The listing builds one solid part. Answer for the finished solid, in the listing's coordinates (mm). Round coordinates to 2 decimals unless told otherwise and drop trailing zeros. Loops run counter-clockwise (first coordinate to the right, second up) from the corner with the lowest first, then second, coordinate; pieces in that order, holes last. Notation, with made-up numbers: (-2.75, 47) -> (11.25, 47) arc R23 ccw to (11.25, 62) -> close; hole circle Ø8 at (27.25, -17.5). An arc over 180 degrees is marked (long way). Answer in a Markdown table with one row per item. Add a question column.
```python
from build123d import *

# Parameters (mm, degrees)
SKETCH_2_R      = 1.75
SKETCH_2_W      = 27.3
SKETCH_2_H      = 20.5
SKETCH_2_W_2    = 9
SKETCH_2_H_2    = 14
EXTRUDE_1_DEPTH = 1.6


with BuildPart() as part:
    # 草图2 → 凸台-拉伸1 (new body)
    with BuildSketch(Plane.XY):
        with BuildLine():
            Line((137.6194709, 153.362234659), (251.6194709, 153.362234659))
            ThreePointArc((251.6194709, 153.362234659), (253.740791244, 152.483555002), (254.6194709, 150.362234659))
            Line((254.6194709, 150.362234659), (254.6194709, 97.362234659))
            ThreePointArc((254.6194709, 97.362234659), (253.740791244, 95.240914315), (251.6194709, 94.362234659))
            Line((251.6194709, 94.362234659), (137.6194709, 94.362234659))
            ThreePointArc((137.6194709, 94.362234659), (135.498150556, 95.240914315), (134.6194709, 97.362234659))
            Line((134.6194709, 97.362234659), (134.6194709, 150.362234659))
            ThreePointArc((134.6194709, 150.362234659), (135.498150556, 152.483555002), (137.6194709, 153.362234659))
        make_face()
        with Locations((139.6194709, 99.362234659)):
            Circle(SKETCH_2_R, mode=Mode.SUBTRACT)
        with Locations((249.6194709, 99.362234659)):
            Circle(SKETCH_2_R, mode=Mode.SUBTRACT)
        with Locations((249.6194709, 148.362234659)):
            Circle(SKETCH_2_R, mode=Mode.SUBTRACT)
        with Locations((139.6194709, 148.362234659)):
            Circle(SKETCH_2_R, mode=Mode.SUBTRACT)
        with Locations((173.2694709, 135.112234659)):
            Rectangle(SKETCH_2_W, SKETCH_2_H, mode=Mode.SUBTRACT)
        with BuildLine():
            Line((211.624069471, 144.588100568), (235.624069471, 144.588100568))
            ThreePointArc((235.624069471, 144.588100568), (236.874069471, 143.338100568), (235.624069471, 142.088100568))
            Line((235.624069471, 142.088100568), (211.624069471, 142.088100568))
            ThreePointArc((211.624069471, 142.088100568), (210.374069471, 143.338100568), (211.624069471, 144.588100568))
        make_face(mode=Mode.SUBTRACT)
        with BuildLine():
            Line((212.067868177, 135.739898553), (236.067868177, 135.739898553))
            ThreePointArc((236.067868177, 135.739898553), (237.317868177, 134.489898553), (236.067868177, 133.239898553))
            Line((236.067868177, 133.239898553), (212.067868177, 133.239898553))
            ThreePointArc((212.067868177, 133.239898553), (210.817868177, 134.489898553), (212.067868177, 135.739898553))
        make_face(mode=Mode.SUBTRACT)
        with BuildLine():
            Line((212.536781854, 118.268660205), (236.536781854, 118.268660205))
            ThreePointArc((236.536781854, 118.268660205), (237.786781854, 117.018660205), (236.536781854, 115.768660205))
            Line((236.536781854, 115.768660205), (212.536781854, 115.768660205))
            ThreePointArc((212.536781854, 115.768660205), (211.286781854, 117.018660205), (212.536781854, 118.268660205))
        make_face(mode=Mode.SUBTRACT)
        with BuildLine():
            Line((150.12910228, 109.191368081), (174.12910228, 109.191368081))
            ThreePointArc((174.12910228, 109.191368081), (175.37910228, 107.941368081), (174.12910228, 106.691368081))
            Line((174.12910228, 106.691368081), (150.12910228, 106.691368081))
            ThreePointArc((150.12910228, 106.691368081), (148.87910228, 107.941368081), (150.12910228, 109.191368081))
        make_face(mode=Mode.SUBTRACT)
        with BuildLine():
            Line((181.33094074, 109.046397883), (205.33094074, 109.046397883))
            ThreePointArc((205.33094074, 109.046397883), (206.58094074, 107.796397883), (205.33094074, 106.546397883))
            Line((205.33094074, 106.546397883), (181.33094074, 106.546397883))
            ThreePointArc((181.33094074, 106.546397883), (180.08094074, 107.796397883), (181.33094074, 109.046397883))
        make_face(mode=Mode.SUBTRACT)
        with BuildLine():
            Line((217.663513674, 108.782143694), (241.663513674, 108.782143694))
            ThreePointArc((241.663513674, 108.782143694), (242.913513674, 107.532143694), (241.663513674, 106.282143694))
            Line((241.663513674, 106.282143694), (217.663513674, 106.282143694))
            ThreePointArc((217.663513674, 106.282143694), (216.413513674, 107.532143694), (217.663513674, 108.782143694))
        make_face(mode=Mode.SUBTRACT)
        with BuildLine():
            Line((218.628069565, 127.463512498), (242.628069565, 127.463512498))
            ThreePointArc((242.628069565, 127.463512498), (243.878069565, 126.213512498), (242.628069565, 124.963512498))
            Line((242.628069565, 124.963512498), (218.628069565, 124.963512498))
            ThreePointArc((218.628069565, 124.963512498), (217.378069565, 126.213512498), (218.628069565, 127.463512498))
        make_face(mode=Mode.SUBTRACT)
        with BuildLine():
            Line((170.018702634, 117.960710868), (194.018702634, 117.960710868))
            ThreePointArc((194.018702634, 117.960710868), (195.268702634, 116.710710868), (194.018702634, 115.460710868))
            Line((194.018702634, 115.460710868), (170.018702634, 115.460710868))
            ThreePointArc((170.018702634, 115.460710868), (168.768702634, 116.710710868), (170.018702634, 117.960710868))
        make_face(mode=Mode.SUBTRACT)
        with BuildLine():
            Line((197.316536613, 102.501223257), (221.316536613, 102.501223257))
            ThreePointArc((221.316536613, 102.501223257), (222.566536613, 101.251223257), (221.316536613, 100.001223257))
            Line((221.316536613, 100.001223257), (197.316536613, 100.001223257))
            ThreePointArc((197.316536613, 100.001223257), (196.066536613, 101.251223257), (197.316536613, 102.501223257))
        make_face(mode=Mode.SUBTRACT)
        with Locations((151.1194709, 138.362234659)):
            Rectangle(SKETCH_2_W_2, SKETCH_2_H_2, mode=Mode.SUBTRACT)
    extrude(amount=EXTRUDE_1_DEPTH)


solid = part.part
```
Item 1: Section B-B, the plane y = 140 is taken. Write down the section's boundary in (x, z).
Item 2: A flat-ended cylindrical pin translates along its axis: P1, Ø2, axis at x = 139.62, y = 148.36, coming from the +Z side. Find the tip coordinate at first contact, or state that the pin passes through.
Item 3: Section A-A, the plane x = 191 is taken. Write down the section's boundary in (y, z), and give its area (3 significant figures).
Item 4: Consider L1, parallel to Y at x = 238.5, z = 0.55; L2, parallel to Y at x = 177.5, z = 0.8; L3, parallel to Y at x = 225, z = 0.95. Determine where each line is inside the solid, lowest interval first. Write a range as from..to.
Item 5: The mould has two halves that part along X. Classify faces 1 (the cylindrical face through (138.33, 149.545, 0.789)), 2 (the cylindrical face through (253.717, 152.507, 0.789)), 3 (the cylindrical face through (135.475, 152.46, 0.789)), 4 (the cylindrical face through (247.87, 99.44, 0.79)): +X half, -X half, draft (parallel to the pull), parting line (faces both ways), or undercut.
Item 6: Section C-C, the plane z = 0.25 is taken. Give the number of separate pieces and of enclosed holes in the cut face, and give its area (3 significant figures).
Here are the results:
| question | item | result |
|---|---|---|
| 1 | outline | (134.62, 0) -> (146.62, 0) -> (146.62, 1.6) -> (134.62, 1.6) -> close; (155.62, 0) -> (159.62, 0) -> (159.62, 1.6) -> (155.62, 1.6) -> close; (186.92, 0) -> (254.62, 0) -> (254.62, 1.6) -> (186.92, 1.6) -> close |
| 2 | P1 | passes through |
| 3 | outline | (94.36, 0) -> (106.55, 0) -> (106.55, 1.6) -> (94.36, 1.6) -> close; (109.05, 0) -> (115.46, 0) -> (115.46, 1.6) -> (109.05, 1.6) -> close; (117.96, 0) -> (153.36, 0) -> (153.36, 1.6) -> (117.96, 1.6) -> close |
| 3 | area | 86.4 mm² |
| 4 | L1 | y = 94.36..106.28, 108.78..124.96, 127.46..153.36 |
| 4 | L2 | y = 94.36..115.46, 117.96..124.86, 145.36..153.36 |
| 4 | L3 | y = 94.36..106.28, 108.78..115.77, 118.27..124.96, 127.46..133.24, 135.74..142.09, 144.59..153.36 |
| 5 | face 1 | undercut |
| 5 | face 2 | +X half |
| 5 | face 3 | -X half |
| 5 | face 4 | undercut |
| 6 | separate pieces | 1 |
| 6 | enclosed holes | 15 |
| 6 | area | 5,760 mm² |
